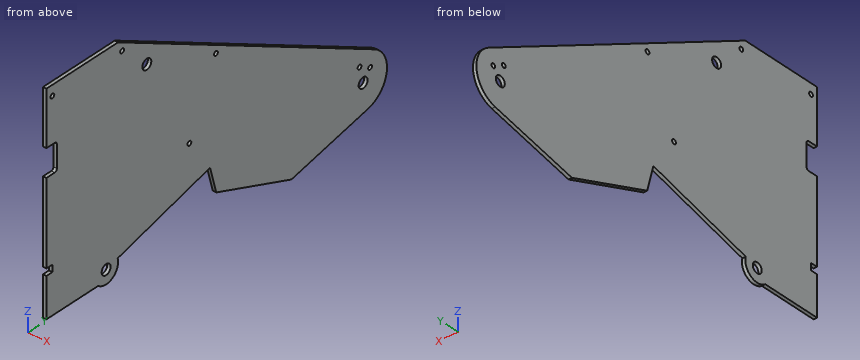
```python
from build123d import *

# Parameters (mm, degrees)
BOSS_EXTRUDE1_DEPTH     = 3.175
SKETCH2_W               = 6.35
SKETCH2_H               = 6.35
CUT_EXTRUDE1_DEPTH      = 413.028889309
F_3_8_CLEARANCE_HOLE1_D = 9.525
SKETCH6_R               = 4.7625
CUT_EXTRUDE2_DEPTH      = 413.028889309
SKETCH10_R              = 2.032
CUT_EXTRUDE4_DEPTH      = 413.028889309
SKETCH11_R              = 2.032
CUT_EXTRUDE5_DEPTH      = 413.028889309
SKETCH13_R              = 2.032
CUT_EXTRUDE6_DEPTH      = 413.028889309
SKETCH14_R              = 2.032
CUT_EXTRUDE7_DEPTH      = 413.028889309


with BuildPart() as part:
    # Sketch1 → Boss-Extrude1 (new body)
    with BuildSketch(Plane(origin=(0, 0, 0), x_dir=(0, 0, -1), z_dir=(1, 0, 0))):
        with BuildLine():
            Line((0, 0), (0, 55.099739587))
            ThreePointArc((0, 55.099739587), (1.26919911, 70.191432251), (-12.812001873, 75.767257994))
            Line((-12.812001873, 75.767257994), (-39.108016855, 173.905321945))
            Line((-39.108016855, 173.905321945), (-14.573500867, 180.47932569))
            Line((-14.573500867, 180.47932569), (15.875, 260.35))
            Line((15.875, 260.35), (-2.186548672, 342.033868455))
            ThreePointArc((-2.186548672, 342.033868455), (-23.459772132, 361.703829452), (-49.323139542, 348.644594092))
            Line((-49.323139542, 348.644594092), (-196.85, 76.2))
            Line((-196.85, 76.2), (-196.85, 0))
            Line((-196.85, 0), (0, 0))
        make_face()
    extrude(amount=BOSS_EXTRUDE1_DEPTH)

    # Sketch2 → Cut-Extrude1 (cut, through all)
    with BuildSketch(Plane(origin=(3.175, 0, 0), x_dir=(0, 0, -1), z_dir=(1, 0, 0))):
        with BuildLine():
            Line((-146.05, 8.790931394), (-146.05, 0))
            Line((-146.05, 0), (-120.65, 0))
            Line((-120.65, 0), (-120.65, 8.790931394))
            ThreePointArc((-120.65, 8.790931394), (-121.349311849, 10.479219545), (-123.0376, 11.178531394))
            Line((-123.0376, 11.178531394), (-143.6624, 11.178531394))
            ThreePointArc((-143.6624, 11.178531394), (-145.350688151, 10.479219545), (-146.05, 8.790931394))
        make_face()
        with Locations((-40.225422327, 3.175)):
            Rectangle(SKETCH2_W, SKETCH2_H)
        with Locations((-226.474577673, 3.175)):
            Rectangle(SKETCH2_W, SKETCH2_H)
    extrude(amount=-CUT_EXTRUDE1_DEPTH, mode=Mode.SUBTRACT)

    # 3/8 Clearance Hole1 (through all)
    with Locations(Plane(origin=(3.175, 0, 0), x_dir=(0, 0, -1), z_dir=(1, 0, 0))):
        with Locations((-26.9875, 336.55), (-9.525, 63.5)):
            Hole(F_3_8_CLEARANCE_HOLE1_D / 2)

    # Sketch6 → Cut-Extrude2 (cut, through all)
    with BuildSketch(Plane(origin=(3.175, 0, 0), x_dir=(0, 0, -1), z_dir=(1, 0, 0))):
        with Locations((-162.275586362, 106.71087433)):
            Circle(SKETCH6_R)
    extrude(amount=-CUT_EXTRUDE2_DEPTH, mode=Mode.SUBTRACT)

    # Sketch10 → Cut-Extrude4 (cut, through all)
    with BuildSketch(Plane(origin=(3.175, 0, 0), x_dir=(0, 0, -1), z_dir=(1, 0, 0))):
        with Locations((-71.256645538, 151.942863158)):
            Circle(SKETCH10_R)
    extrude(amount=-CUT_EXTRUDE4_DEPTH, mode=Mode.SUBTRACT)

    # Sketch11 → Cut-Extrude5 (cut, through all)
    with BuildSketch(Plane(origin=(3.175, 0, 0), x_dir=(0, 0, -1), z_dir=(1, 0, 0))):
        with Locations((-187.325, 80.45454267)):
            Circle(SKETCH11_R)
        with Locations((-187.325, 6.35)):
            Circle(SKETCH11_R)
    extrude(amount=-CUT_EXTRUDE5_DEPTH, mode=Mode.SUBTRACT)

    # Sketch13 → Cut-Extrude6 (cut, through all)
    with BuildSketch(Plane.ZY):
        with Locations((36.31904262, 343.988077457)):
            Circle(SKETCH13_R)
        with Locations((42.366339666, 332.820257685)):
            Circle(SKETCH13_R)
    extrude(amount=-CUT_EXTRUDE6_DEPTH, mode=Mode.SUBTRACT)

    # Sketch14 → Cut-Extrude7 (cut, through all)
    with BuildSketch(Plane(origin=(3.175, 0, 0), x_dir=(0, 0, -1), z_dir=(1, 0, 0))):
        with Locations((-133.35, 180.132641428)):
            Circle(SKETCH14_R)
    extrude(amount=-CUT_EXTRUDE7_DEPTH, mode=Mode.SUBTRACT)


solid = part.part
```
Read the model definition and answer for the solid it produces. Units are mm, in the model's axes. Coordinates: 2 decimals unless noted, no trailing zeros. Loops run counter-clockwise (first coordinate to the right, second up) from the corner with the lowest first, then second, coordinate; pieces in that order, holes last.
(1) Flat-ended cylindrical pins translate along their axes: pin 1 Ø1.6 at (x, z) = (1.5, 137) entering from -Y; pin 2 Ø2 at (y, z) = (262, 69.5) entering from -X; pin 3 Ø8.5 at (y, z) = (63.5, 9.525) entering from +X. Find the tip coordinate at first contact, or state that the pin passes through.
Solution:
pin 1: stops at y = 11.18
pin 2: stops at x = 0
pin 3: passes through
(2) The part is cut by section D-D (z = 98.5). Determine the outline of the cut face in (x, y) (3 decimals).
Solution:
outline: (0, 0) - (3.175, 0) - (3.175, 257.827) - (0, 257.827) - close
(3) Consider line 1 along Y through (x, z) = (1.65, 158); line 2 along Z through (x, y) = (2.15, 25.5); line 3 along Z through (x, y) = (0.9, 80.5). Determine where each line is inside the solid, lowest interval first.
Solution:
line 1: y = 0 to 104.61, 108.81 to 147.95
line 2: z = 0 to 196.85
line 3: z = 14.08 to 185.29, 189.36 to 194.52
(4) The part is cut by section B-B (x = 1). Count the separate pieces of the cut face and the enclosed holes in it, and give its area (3 significant figures).
Solution:
separate pieces: 1
enclosed holes: 9
area: 46,200 mm2
(5) The part is cut by section C-C (y = 23.5). Determine the outline of the cut face in (x, z) (3 decimals).
Solution:
outline: (0, 0) - (3.175, 0) - (3.175, 196.85) - (0, 196.85) - close
